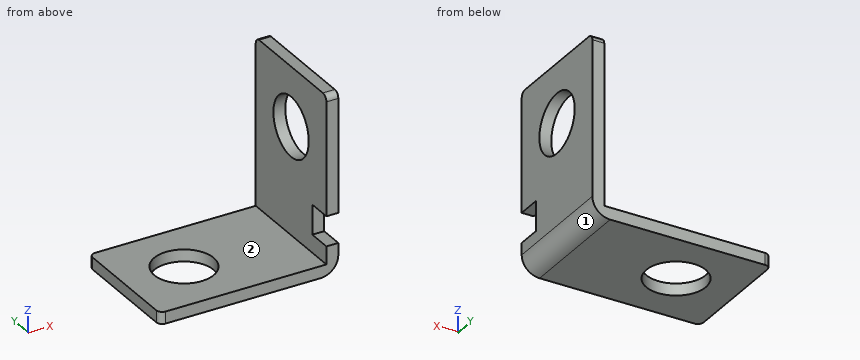
```python
from build123d import *

# Parameters (mm, degrees)
F1_DEPTH = 20
F2_R     = 5
F3_DEPTH = 2.001
F4_R     = 5
F5_DEPTH = 2.001
F6_W     = 4
F6_H     = 5
F7_DEPTH = 30.001
F8_R     = 1


with BuildPart() as f1:
    # F0 (on Front) → F1 (new body)
    with BuildSketch(Plane.XZ):
        with BuildLine():
            Line((0, 2), (0, 0))
            Line((0, 0), (27, 0))
            ThreePointArc((27, 0), (29.12132, 0.87868), (30, 3))
            Line((30, 3), (30, 30))
            Line((30, 30), (28, 30))
            Line((28, 30), (28, 2))
            Line((28, 2), (0, 2))
        make_face()
    extrude(amount=F1_DEPTH)

    # F2 (on face) → F3 (cut, through all)
    with BuildSketch(Plane(origin=(28, 0, 0), x_dir=(0, -1, 0), z_dir=(-1, 0, 0))):
        with Locations((10, 20)):
            Circle(F2_R)
    extrude(amount=-F3_DEPTH, mode=Mode.SUBTRACT)

    # F4 (on face) → F5 (cut, through all)
    with BuildSketch(Plane.XY.offset(2)):
        with Locations((10, -10)):
            Circle(F4_R)
    extrude(amount=-F5_DEPTH, mode=Mode.SUBTRACT)

    # F6 (on face) → F7 (cut, through all)
    with BuildSketch(Plane.YZ.offset(30)):
        with Locations((-18, 7.5)):
            Rectangle(F6_W, F6_H)
    extrude(amount=-F7_DEPTH, mode=Mode.SUBTRACT)

    # F8
    f8_edges = [f1.edges().sort_by_distance(p)[0] for p in [
        (0, -20, 1),
        (0, 0, 1),
        (29, 0, 30),
        (29, -20, 30),
    ]]
    fillet(f8_edges, radius=F8_R)


solid = f1.part
```
Model file for the job. Use its own axes, mm. Face numbers are marked on the shaded views. A direction names the side the tool comes from. Coordinates: 2 decimals unless noted, no trailing zeros. Loops run counter-clockwise (first coordinate to the right, second up) from the corner with the lowest first, then second, coordinate; pieces in that order, holes last. Notation, with made-up numbers: (50, 15.25) - (84, 15.25) arc R26 ccw to (84, 37.25) - close; hole circle Ø2 at (42.25, -8). An arc over 180 degrees is marked (long way). Answer as a JSON object with one key per item and string values. Group by question number.
(1) Cut at D-D (y = -6). Give the cut face in (x, z), then the cut area to 3 significant figures.
(2) Cut at B-B (y = -10). Give the cut face in (x, z), then the cut area to 3 significant figures.
(3) Cut at A-A (x = 10). Give the cut face in (y, z).
(4) Cut at C-C (z = 22.5). Give the cut face in (x, y).
(5) Probe line 1 along Y through (x, z) = (10, 1.45); line 2 along Z through (x, y) = (22.5, -13.25); line 3 along X through (y, z) = (-14, 16.75). List the from-to ranges inside material, lowest first.
(6) Flat gauge pins, fed straight in: pin 1 (0.6 mm diameter, centred on x = 29, z = 7.5, fed in from -Y); pin 2 (8 mm diameter, centred on y = -10, z = 20, fed in from -X); pin 3 (1.5 mm diameter, centred on x = 6, y = -3.5, fed in from +Z); pin 4 (1 mm diameter, centred on x = 29.5, y = -18.5, fed in from -Z). Where does each tip first touch, or does it go through?
(7) Tool access for the marked faces 1 and 2: list every direction of +Z, -Z, +X, -X, +Y, -Y with a clear straight run to the whole face (end or side of a thin tool).
Geometry says:
{
 "1": {"outline": "(0, 0) - (7, 0) - (7, 2) - (0, 2) - close; (13, 0) - (27, 0) arc R3 ccw to (30, 3) - (30, 17) - (28, 17) - (28, 2) - (13, 2) - close; (28, 23) - (30, 23) - (30, 30) - (28, 30) - close", "area": "90.1 mm^2"},
 "2": {"outline": "(0, 0) - (5, 0) - (5, 2) - (0, 2) - close; (15, 0) - (27, 0) arc R3 ccw to (30, 3) - (30, 15) - (28, 15) - (28, 2) - (15, 2) - close; (28, 25) - (30, 25) - (30, 30) - (28, 30) - close", "area": "74.1 mm^2"},
 "3": {"outline": "(-20, 0) - (-15, 0) - (-15, 2) - (-20, 2) - close; (-5, 0) - (0, 0) - (0, 2) - (-5, 2) - close"},
 "4": {"outline": "(28, -20) - (30, -20) - (30, -14.33) - (28, -14.33) - close; (28, -5.67) - (30, -5.67) - (30, 0) - (28, 0) - close"},
 "5": {"line 1": "y = -20 to -15, -5 to 0", "line 2": "z = 0 to 2", "line 3": "x = 28 to 30"},
 "6": {"pin 1": "stops at y = -16", "pin 2": "passes through", "pin 3": "stops at z = 2", "pin 4": "stops at z = 0.76"},
 "7": {"face 1": "-Z, +X, +Y, -Y", "face 2": "+Z, -X, +Y, -Y"}
}
